For this review, take the finished solid that the model builds, in its own axes (mm). Face numbers are marked on the shaded views. A direction names the side the tool comes from. Coordinates: 2 decimals unless noted, no trailing zeros. Order: outer loops, then holes, each group sorted by start corner. A loop starts at its lowest first (then second) coordinate and runs counter-clockwise, first axis right, second up. Notation, with made-up numbers: (-28.75, 51.5) -> (25.25, 51.5) arc R37 ccw to (25.25, 90.5) -> close; hole circle Ø5 at (82.25, 16.5). An arc over 180 degrees is marked (long way). Answer as a JSON object with one key per item and string values. Group by question number.
1) For pin 1 (14 mm diameter, centred on x = -2, y = 1, fed in from +Z); pin 2 (4.5 mm diameter, centred on x = -15, z = 75, fed in from -Y); pin 3 (10 mm diameter, centred on x = 6.5, z = 26.5, fed in from -Y), all flat-tipped, find the tip position at first contact; note any pin that passes through.
2) Add section A-A, the plane z = 44. Write out the cut boundary in (x, y).
3) Add section C-C, the plane x = -12.5. Write out the cut boundary in (y, z), then the cut area to 3 significant figures.
4) Wall thickness on L1, parallel to Z at x = -15, y = 25; L2, parallel to X at y = 26.7, z = 75; L3, parallel to Z at x = 6.5, y = -2.5: over which ranges is each line inside the solid? List them lowest first.
5) Add section D-D, the plane y = 10.5. Write out the cut boundary in (x, z).
6) Machinability: for the marked faces 1 and 2, which of the approach directions +Z, -Z, +X, -X, +Y, -Y give a long, thin tool a straight path to every point of the face, cutting with its end or side? Answer none if there is none.
7) Add section B-B, the plane y = -15. Write out the cut boundary in (x, z), then the cut area to 3 significant figures.
from build123d import *

# Parameters (mm, degrees)
F0_W     = 60
F0_H     = 60
F0_R     = 1.95
F1_DEPTH = 4
F2_W     = 60
F2_H     = 86
F2_R     = 1.45
F3_DEPTH = 6
F5_DEPTH = 60


with BuildPart() as f1:
    # F0 (on Top) → F1 (new body)
    with BuildSketch(Plane.XY):
        Rectangle(F0_W, F0_H)
        with Locations((-16, -15)):
            Circle(F0_R, mode=Mode.SUBTRACT)
        with Locations((16, -15)):
            Circle(F0_R, mode=Mode.SUBTRACT)
        with Locations((-16, 5)):
            Circle(F0_R, mode=Mode.SUBTRACT)
        with Locations((16, 5)):
            Circle(F0_R, mode=Mode.SUBTRACT)
    extrude(amount=F1_DEPTH)

    # F2 (on face) → F3 (join)
    with BuildSketch(Plane(origin=(0, 30, 0), x_dir=(-1, 0, 0), z_dir=(0, 1, 0))):
        with Locations((0, 47)):
            Rectangle(F2_W, F2_H)
        with Locations((-15, 44)):
            Circle(F2_R, mode=Mode.SUBTRACT)
        with Locations((15, 44)):
            Circle(F2_R, mode=Mode.SUBTRACT)
        with Locations((-15, 75)):
            Circle(F2_R, mode=Mode.SUBTRACT)
        with Locations((15, 75)):
            Circle(F2_R, mode=Mode.SUBTRACT)
    extrude(amount=-F3_DEPTH)

    # F4 (on face) → F5 (join)
    with BuildSketch(Plane.YZ.offset(30)):
        Polygon((24, 34.079062), (16.5, 4), (24, 4), align=None)
    extrude(amount=-F5_DEPTH)


solid = f1.part
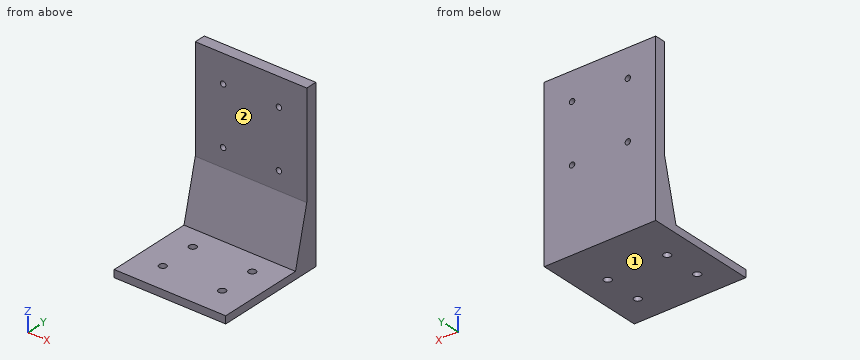
Output values:
{
 "1": {"pin 1": "stops at z = 4", "pin 2": "stops at y = 24", "pin 3": "stops at y = 20.86"},
 "2": {"outline": "(-30, 24) -> (-16.45, 24) -> (-16.45, 30) -> (-30, 30) -> close; (-13.55, 24) -> (13.55, 24) -> (13.55, 30) -> (-13.55, 30) -> close; (16.45, 24) -> (30, 24) -> (30, 30) -> (16.45, 30) -> close"},
 "3": {"outline": "(-30, 0) -> (30, 0) -> (30, 90) -> (24, 90) -> (24, 34.08) -> (16.5, 4) -> (-30, 4) -> close", "area": "869 mm²"},
 "4": {"L1": "z = 0 to 42.55, 45.45 to 73.55, 76.45 to 90", "L2": "x = -30 to -16.45, -13.55 to 13.55, 16.45 to 30", "L3": "z = 0 to 4"},
 "5": {"outline": "(-30, 0) -> (30, 0) -> (30, 4) -> (-30, 4) -> close"},
 "6": {"face 1": "-Z, +X, -X, +Y, -Y", "face 2": "+Z, +X, -X, -Y"},
 "7": {"outline": "(-30, 0) -> (-17.95, 0) -> (-17.95, 4) -> (-30, 4) -> close; (-14.05, 0) -> (14.05, 0) -> (14.05, 4) -> (-14.05, 4) -> close; (17.95, 0) -> (30, 0) -> (30, 4) -> (17.95, 4) -> close", "area": "209 mm²"}
}
